```python
from build123d import *

# Parameters (mm, degrees)
F1_DEPTH = 150
F2_R     = 2


with BuildPart() as f1:
    # F0 (on Right) → F1 (new body)
    with BuildSketch(Plane.YZ):
        Polygon((200, 0), (0, 0), (0, -15), (-15, -15), (-15, -30), (-30, -30), (-30, -45), (-45, -45), (-45, -60), (-60, -60), (-60, -75), (200, -75), align=None)
    extrude(amount=F1_DEPTH)

    # F2
    f2_edges = [f1.edges().sort_by_distance(p)[0] for p in [
        (75, -15, -15),
        (75, 0, 0),
        (75, -30, -30),
        (75, -45, -45),
        (75, -60, -60),
    ]]
    fillet(f2_edges, radius=F2_R)


solid = f1.part
```
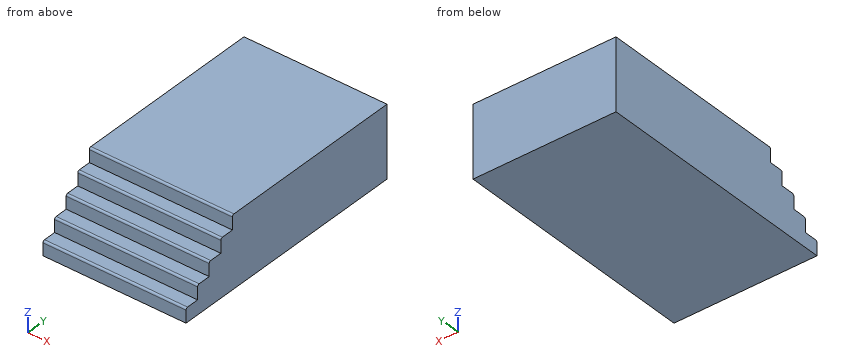
CAD build for the part. Positions are in the model's coordinates, mm. Round coordinates to 2 decimals unless told otherwise and drop trailing zeros. Loops run counter-clockwise (first coordinate to the right, second up) from the corner with the lowest first, then second, coordinate; pieces in that order, holes last. Notation, with made-up numbers: M 45.25,36 L 52.25,36 A15 ccw 52.25,54 Z; hole C 29.25,-3 d4. An arc over 180 degrees is marked long. Return JSON: item names as keys, results as strings. Group by question number.
(1) Saw through at A-A, the plane x = 90.5. List the corners of the cut face in (y, z).
(2) Saw through at C-C, the plane z = -57.5. List the corners of the cut face in (x, y).
(3) Wall check: probe 1 along Z at (x, y) = (116.5, -9); probe 2 along Y at (x, z) = (92.5, -10.5); probe 3 along Y at (x, z) = (113, -24.5). Give the ranges that are in metal, low to high. Write a range as [from, to].
(4) Drop flat-ended pins along their axis: P1, Ø14.5, axis at x = 42, y = -19, coming from the +Z side; P2, Ø4, axis at x = 131.5, z = -17.5, coming from the -Y side; P3, Ø14.5, axis at x = 38, z = -40, coming from the -Y side. Give the stop position or say it passes through.
(5) Saw through at B-B, the plane z = -35. List the corners of the cut face in (x, y).
Answer list:
{
 "1": {"outline": "M -60,-75 L 200,-75 L 200,0 L 2,0 A2 ccw 0,-2 L 0,-15 L -13,-15 A2 ccw -15,-17 L -15,-30 L -28,-30 A2 ccw -30,-32 L -30,-45 L -43,-45 A2 ccw -45,-47 L -45,-60 L -58,-60 A2 ccw -60,-62 Z"},
 "2": {"outline": "M 0,-45 L 150,-45 L 150,200 L 0,200 Z"},
 "3": {"probe 1": "[-75, -15]", "probe 2": "[0, 200]", "probe 3": "[-15, 200]"},
 "4": {"P1": "z = -15", "P2": "y = -15", "P3": "y = -45"},
 "5": {"outline": "M 0,-30 L 150,-30 L 150,200 L 0,200 Z"}
}
